Part print with two shaded views. Sizes in mm from the minimum x, y, z corner. A direction names the side the tool comes from. Give positions to 0.01 mm unless a question says otherwise; leave off trailing zeros. Loops run counter-clockwise (first coordinate to the right, second up) from the corner with the lowest first, then second, coordinate; pieces in that order, holes last. Notation, with made-up numbers: M 5,28.25 L 12,28.25 A26 cw 12,63.25 Z; hole C 40.5,13 d8. An arc over 180 degrees is marked long. Answer in a Markdown table with one row per item.
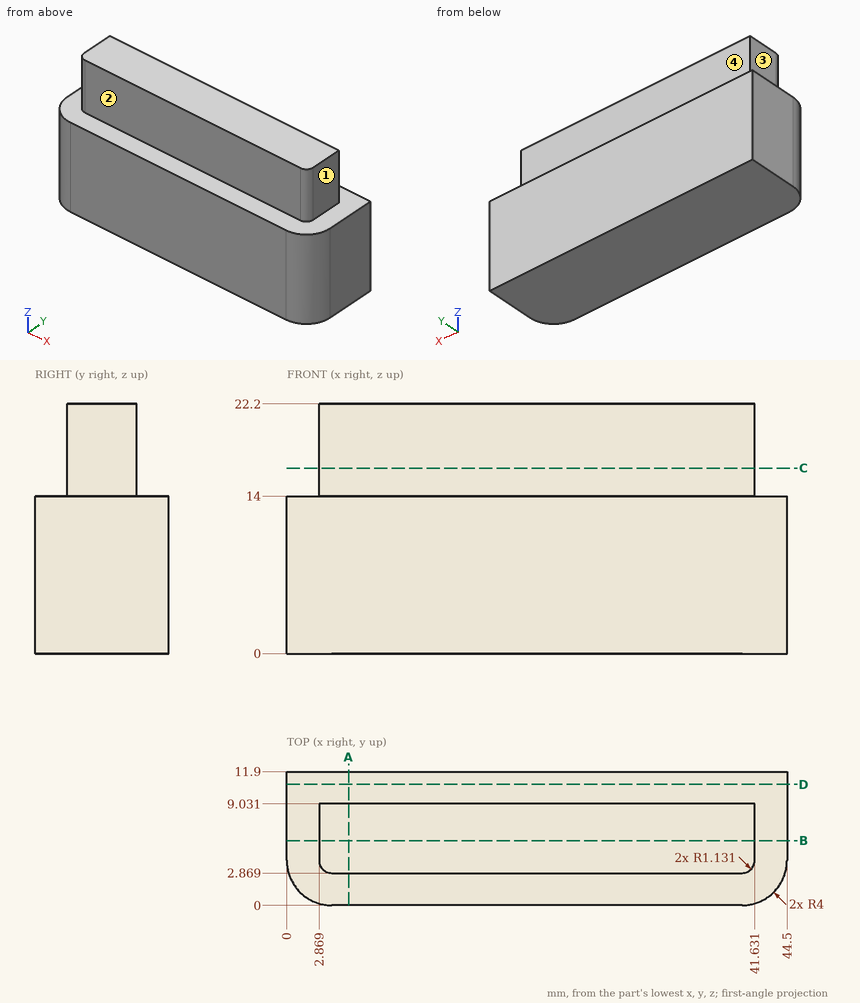
Q1. Saw through at C-C (z = 16.5). Give the cut face in (x, y).
Reported:
| item | result |
|---|---|
| outline | M 2.87,4 A1.13 ccw 4,2.87 L 40.5,2.87 A1.13 ccw 41.63,4 L 41.63,9.03 L 2.87,9.03 Z |
Q2. Probe probe 1 along Y at (x, z) = (4.5, 17.5); probe 2 along Z at (x, y) = (27.5, 9.25); probe 3 along Y at (x, z) = (42, 5.25). List the from-to ranges inside material, lowest first.
Reported:
| item | result |
|---|---|
| probe 1 | 2.87 to 9.03 |
| probe 2 | 0 to 14 |
| probe 3 | 0.29 to 11.9 |
Q3. Saw through at D-D (y = 10.75). Give the cut face in (x, z).
Reported:
| item | result |
|---|---|
| outline | M 0,0 L 44.5,0 L 44.5,14 L 0,14 Z |
Q4. Saw through at A-A (x = 5.5). Give the cut face in (y, z), and give its area (3 significant figures).
Reported:
| item | result |
|---|---|
| outline | M 0,0 L 11.9,0 L 11.9,14 L 9.03,14 L 9.03,22.2 L 2.87,22.2 L 2.87,14 L 0,14 Z |
| area | 217 mm² |
Q5. 3-axis set-ups, long thin cutter, end or side, ignore diameter. For the marked faces 1, 2, 3 and 4: which of +Z, -Z, +X, -X, +Y, -Y reach the whole face in a straight line?
Reported:
| item | result |
|---|---|
| face 1 | +Z, +X, +Y, -Y |
| face 2 | +Z, +X, -X, -Y |
| face 3 | +Z, -X, +Y, -Y |
| face 4 | +Z, +X, -X, +Y |
Q6. Saw through at B-B (y = 5.75). Give the cut face in (x, z), and give its area (3 significant figures).
Reported:
| item | result |
|---|---|
| outline | M 0,0 L 44.5,0 L 44.5,14 L 41.63,14 L 41.63,22.2 L 2.87,22.2 L 2.87,14 L 0,14 Z |
| area | 941 mm² |
Q7. Drop flat-ended pins along their axis: pin 1 (4 mm diameter, centred on x = 13.5, z = 19, fed in from -Y); pin 2 (1.5 mm diameter, centred on y = 5.5, z = 18.5, fed in from +X); pin 3 (1.5 mm diameter, centred on y = 6, z = 19, fed in from -X). Give the stop position or say it passes through.
Reported:
| item | result |
|---|---|
| pin 1 | y = 2.87 |
| pin 2 | x = 41.63 |
| pin 3 | x = 2.87 |
